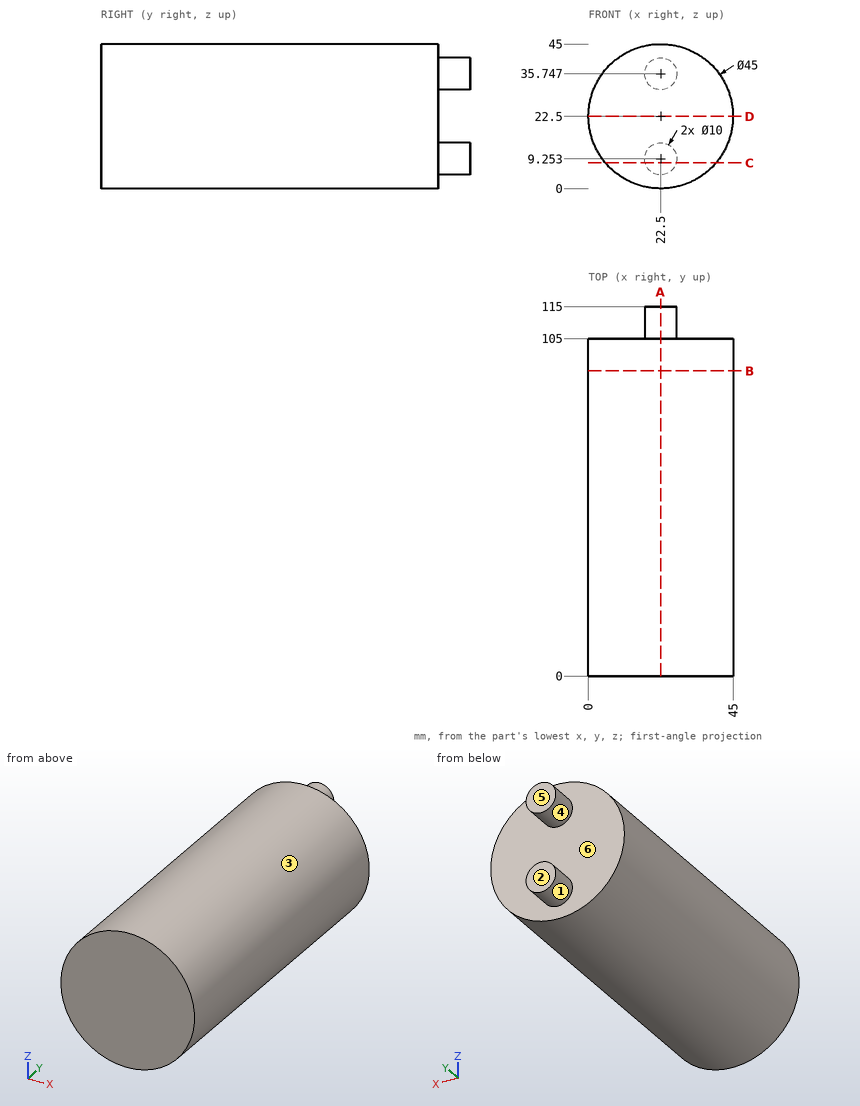
Here's the drawing with two shaded views (mm, measured from the low corner). I have some questions. A direction names the side the tool comes from. Coordinates: 2 decimals unless noted, no trailing zeros. Write each loop counter-clockwise with the first axis right and the second up, starting at its lowest first coordinate (ties: lowest second). Pieces come first, ordered by that corner, then holes. Notation, with made-up numbers: (-17, 30) - (39, 30) arc R10 cw to (39, 48) - close; hole circle Ø8 at (-36, -29). An arc over 180 degrees is marked (long way). Return JSON: item names as keys, results as strings.
Q1. If we section it at C-C (z = 8): Please give me the cut outline in (x, y).
Computed values:
{"outline": "(5.3, 0) - (39.7, 0) - (39.7, 105) - (27.34, 105) - (27.34, 115) - (17.66, 115) - (17.66, 105) - (5.3, 105) - close"}
Q2. Thinking about a two-plate mould opening in Z: for the marked faces 1, 2, 3 and 4, which applies, +Z half, -Z half, draft (parallel to the pull), parting line (faces both ways), or undercut?
Computed values:
{"face 1": "undercut", "face 2": "draft", "face 3": "parting line", "face 4": "undercut"}
Q3. If we section it at B-B (y = 95): Please give me the cut outline in (x, z).
Computed values:
{"outline": "circle Ø45 at (22.5, 22.5)"}
Q4. I'm going to push flat-ended pins straight in: pin 1 Ø1 at (x, z) = (27, 23.5) entering from -Y; pin 2 Ø1.5 at (y, z) = (17, 20) entering from -X; pin 3 Ø8 at (y, z) = (58, 15) entering from -X; pin 4 Ø6 at (x, y) = (12, 82) entering from +Z. Where does each tip first touch, or does it pass through?
Computed values:
{"pin 1": "stops at y = 0", "pin 2": "stops at x = 0.07", "pin 3": "stops at x = 0.27", "pin 4": "stops at z = 43.71"}
Q5. If we section it at A-A (x = 22.5): Please give me the cut outline in (y, z), then the cut area to 4 significant figures.
Computed values:
{"outline": "(0, 0) - (105, 0) - (105, 4.25) - (115, 4.25) - (115, 14.25) - (105, 14.25) - (105, 30.75) - (115, 30.75) - (115, 40.75) - (105, 40.75) - (105, 45) - (0, 45) - close", "area": "4,925 mm2"}
Q6. If we section it at D-D (z = 22.5): Please give me the cut outline in (x, y), then the cut area to 4 significant figures.
Computed values:
{"outline": "(0, 0) - (45, 0) - (45, 105) - (0, 105) - close", "area": "4,725 mm2"}
Q7. Please list where these lines run through material, in increasing order: L1, parallel to Y at x = 30, z = 24.5; L2, parallel to X at y = 30.5, z = 23.5; L3, parallel to Z at x = 23, y = 32.5. Write a range as from..to.
Computed values:
{"L1": "y = 0..105", "L2": "x = 0.02..44.98", "L3": "z = 0.01..44.99"}
Q8. On a 3-axis mill with a long thin cutter (end or side, diameter ignored), from which of +Z, -Z, +X, -X, +Y, -Y can I reach the whole of each face in a straight line? I mean the marked faces 5 and 6. Say none if no direction works.
Computed values:
{"face 5": "+Z, -Z, +X, -X, +Y", "face 6": "+Y"}
